Could you check a few things on this model? Use its own coordinates, in mm. A direction names the side the tool comes from. Give positions to 0.01 mm unless a question says otherwise; leave off trailing zeros. Loops run counter-clockwise (first coordinate to the right, second up) from the corner with the lowest first, then second, coordinate; pieces in that order, holes last. Notation, with made-up numbers: (57, 37.25) - (62, 37.25) arc R6 cw to (62, 42.25) - close; hole circle Ø1 at (10.5, 51.5). An arc over 180 degrees is marked (long way). One line per item, written item: value. Start each with the question number.
Q1. If I drill on line 1 (Y direction, x = 20, z = -2) (3 decimals); line 2 (Y direction, x = 244.5, z = 0); line 3 (Z direction, x = 192, y = -35), over which ranges is the centre line in solid material (lowest first)? Write a range as from..to.
Q2. I want a section at A-A (z = -63.5). Please give me the cut outline in (x, y), then the cut area to 3 significant figures.
Q3. For faces 4 (the face through (234, -2.5, 56)), 5 (the face through (310, -71.5, -23.3)), which set-ups out of +Z, -Z, +X, -X, +Y, -Y let a thin tool reach every point of the face, with its end or its side?
Q4. I'm going to push flat-ended pins straight in: P1, Ø1.5, axis at y = -72, z = -6.5, coming from the +X side; P2, Ø1.7, axis at x = 74.5, y = -72, coming from the -Z side; P3, Ø15, axis at x = 231, z = 66, coming from the +Y side. Where does each tip first touch, or does it pass through?
Q5. I want a section at B-B (y = 22.5). Please give me the cut outline in (x, z), then the cut area to 3 significant figures.
Q6. If we mould it in two halves opening along Y, with no side actions, what happens to faces 1 (the face through (157.17, 66.538, 34.608)), 2 (the face through (0, -71.5, -23.3)), 3 (the face through (157.17, -3.517, -79.923))? For each: released by +Y, released by -Y, zero draft, split by the parting line, or undercut.
Q7. I want a section at C-C (x = 142.5). Please give me the cut outline in (y, z).
Q8. I want a section at D-D (z = -7.5). Please give me the cut outline in (x, y), then the cut area to 3 significant figures.
```python
from build123d import *

# Parameters (mm, degrees)
SKIZZE1_W                            = 310
SKIZZE1_H                            = 5
AUFSATZ_LINEAR_AUSTRAGEN1_DEPTH      = 2.5
AUFSATZ_LINEAR_AUSTRAGEN1_DEPTH_BACK = 2.5
SKIZZE5_W                            = 30
SKIZZE5_H                            = 30
AUFSATZ_LINEAR_AUSTRAGEN2_DEPTH      = 5
DURCHGANGSLOCH_F_R_M51_D             = 5.5
DURCHGANGSLOCH_F_R_M51_DEPTH         = 10


with BuildPart() as part:
    # Skizze1 → Rotation1 (revolve)
    with BuildSketch(Plane.XY, mode=Mode.PRIVATE) as rotation1_sk:
        with Locations((155, 77.5)):
            Rectangle(SKIZZE1_W, SKIZZE1_H)
    revolve(rotation1_sk.sketch.rotate(Axis((0, 0, 0), (1, 0, 0)), 90), axis=Axis((0, 0, 0), (1, 0, 0)))

    # Skizze3 → Aufsatz-Linear austragen1 (add, two sides: drawn at the far end of the back side and taken through both)
    with BuildSketch(Plane(origin=(0, 0, 0), x_dir=(1, 0, 0), z_dir=(0, 1, 0)).offset(-AUFSATZ_LINEAR_AUSTRAGEN1_DEPTH_BACK)):
        Polygon((255, -55), (275, -55), (275, -45), (195, -45), (195, -55), (215, -55), (215, -75), (255, -75), align=None)
    extrude(amount=AUFSATZ_LINEAR_AUSTRAGEN1_DEPTH + AUFSATZ_LINEAR_AUSTRAGEN1_DEPTH_BACK)

    # Skizze5 → Aufsatz-Linear austragen2 (add)
    with BuildSketch(Plane(origin=(0, -75, 0), x_dir=(1, 0, 0), z_dir=(0, 1, 0))):
        with Locations((70, 0)):
            Rectangle(SKIZZE5_W, SKIZZE5_H)
    aufsatz_linear_austragen2 = extrude(amount=AUFSATZ_LINEAR_AUSTRAGEN2_DEPTH)

    # Durchgangsloch für M51
    with Locations(Plane(origin=(0, -70, 0), x_dir=(1, 0, 0), z_dir=(0, 1, 0))):
        with Locations((70, 0)):
            durchgangsloch_f_r_m51 = Hole(DURCHGANGSLOCH_F_R_M51_D / 2, depth=DURCHGANGSLOCH_F_R_M51_DEPTH)

    # Spiegeln2: Aufsatz-Linear austragen2, Durchgangsloch für M51 across plane
    add(aufsatz_linear_austragen2.mirror(Plane.ZY.offset(-155)))
    add(durchgangsloch_f_r_m51.mirror(Plane.ZY.offset(-155)), mode=Mode.SUBTRACT)


solid = part.part
```
Worked answers:
1. line 1: y = -79.975..-74.973, 74.973..79.975
1. line 2: y = -80..-70, 75..80
1. line 3: z = -71.94..-66.33, 66.33..71.94
2. outline: (0, -48.66) - (310, -48.66) - (310, -39.91) - (0, -39.91) - close; (0, 39.91) - (310, 39.91) - (310, 48.66) - (0, 48.66) - close
2. area: 5,430 mm²
3. face 4: +X, -X
3. face 5: +Z, -Z, +X, +Y, -Y
4. P1: stops at x = 255
4. P2: stops at z = -36.57
4. P3: stops at y = 54.57
5. outline: (0, -76.77) - (310, -76.77) - (310, -71.55) - (0, -71.55) - close; (0, 71.55) - (310, 71.55) - (310, 76.77) - (0, 76.77) - close
5. area: 3,240 mm²
6. face 1: undercut
6. face 2: zero draft
6. face 3: split by the parting line
7. outline: circle Ø160 at (0, 0); hole circle Ø150 at (0, 0)
8. outline: (0, -79.65) - (310, -79.65) - (310, -74.62) - (255, -74.62) - (255, -70) - (225, -70) - (225, -74.62) - (85, -74.62) - (85, -70) - (55, -70) - (55, -74.62) - (0, -74.62) - close; (0, 74.62) - (310, 74.62) - (310, 79.65) - (0, 79.65) - close
8. area: 3,390 mm²
